Geometry: final body of the model. Coordinates: model frame, mm. A direction names the side the tool comes from. Round coordinates to 2 decimals unless told otherwise and drop trailing zeros. Write each loop counter-clockwise with the first axis right and the second up, starting at its lowest first coordinate (ties: lowest second). Pieces come first, ordered by that corner, then holes.
from build123d import *

# Parameters (mm, degrees)
F4_D            = 6.096
F4_CBORE_D      = 12.192
F4_CBORE_DEPTH  = 6.096
F4_COPIES_COUNT = 6
F5_R            = 7.3585229381
F6_R            = 8.8302275257
F7_SIZE         = 1.27


# Not quite as in the source:
# - a pattern or mirror of a feature is missing from the dataset's text; its kind, count and spacing are read off the source's solid


with BuildPart() as f2:
    # F1 (on Top) → F2 (revolve)
    with BuildSketch(Plane.XY):
        Polygon((0, 23.1950208545), (0, 0), (19.8225509375, 0), (19.8225509375, 20.0292905793), (51.67459324, 20.0292905793), (51.67459324, 28.776070103), (10.3429872543, 28.776070103), (10.3429872543, 23.1950208545), align=None)
    revolve(axis=Axis((0, 11.5975104272, 0), (0, -1, 0)))

    # F4 (through all)
    with Locations(Plane(origin=(0, 28.776070103, 0), x_dir=(-1, 0, 0), z_dir=(0, 1, 0))):
        with Locations((0, -38.1)):
            f4 = CounterBoreHole(F4_D / 2, F4_CBORE_D / 2, F4_CBORE_DEPTH)

    # F4_copies: F4 ×6 about axis
    f4_copies_axis = Axis((0, 0, 0), (0, 1, 0))
    for i in range(1, F4_COPIES_COUNT):
        add(f4.rotate(f4_copies_axis, i * 360 / F4_COPIES_COUNT), mode=Mode.SUBTRACT)

    # F5
    f5_edges = [f2.edges().sort_by_distance(p)[0] for p in [
        (-19.822551, 20.029291, 0),
    ]]
    fillet(f5_edges, radius=F5_R)

    # F6
    f6_edges = [f2.edges().sort_by_distance(p)[0] for p in [
        (-19.822551, 0, 0),
    ]]
    fillet(f6_edges, radius=F6_R)

    # F7
    f7_edges = [f2.edges().sort_by_distance(p)[0] for p in [
        (-51.674593, 20.029291, 0),
        (-51.674593, 28.77607, 0),
    ]]
    chamfer(f7_edges, length=F7_SIZE)


solid = f2.part
1) Section B-B on y = 26.25. Output: boundary loops of the cut face in (x, z), plus the area to 3 significant figures.
2) Section C-C on x = 0. State how many separate pieces and enclosed holes the cut face has, plus the area to 3 significant figures.
3) Line query: probe 1 along Z at (x, y) = (0, 21.8); probe 2 along Z at (x, y) = (0, 26.5); probe 3 along Z at (x, y) = (30, 25.5). Output: solid intervals per line, ascending.
4) Draft query along Z for faces 1 (the cylindrical face through (49.29, 24.45, 15.52)), 2 (the flat face through (-22, 20.029, -22)), 3 (the cylindrical face through (-38.81, 25.77, 20.88)). Return one class per face: pulls with the +Z half, pulls with the -Z half, needs draft (parallel to the pull), parting line crosses it, or undercut.
5) First-contact query: P1, Ø10, axis at x = -25, z = 25.5, coming from the -Y side; P2, Ø12, axis at y = 21.5, z = -28.5, coming from the +X side; P3, Ø6, axis at x = 30.5, z = -20.5, coming from the +Y side. Flat tips, straight axial feed; report the tip coordinate or a pass-through.
6) Reachability of faces 4 (the cylindrical face through (10.66, 10.78, 16.71)), 5 (the flat face through (0, 0, 0)), 6 (the flat face through (30, 22.68, 21)) from +Z, -Z, +X, -X, +Y, -Y: full face, straight path, thin tool, end or side. Return the list, or none.
7) Section A-A on z = 0. Output: boundary loops of the cut face in (x, y).
Filled in:
1. outline: circle Ø103.35 at (0, 0); hole circle Ø12.19 at (-33, -19.05); hole circle Ø12.19 at (-33, 19.05); hole circle Ø20.69 at (0, 0); hole circle Ø12.19 at (0, -38.1); hole circle Ø12.19 at (0, 38.1); hole circle Ø12.19 at (33, -19.05); hole circle Ø12.19 at (33, 19.05)
1. area: 7,350 mm2
2. separate pieces: 3
2. enclosed holes: 0
2. area: 1,390 mm2
3. probe 1: z = -51.67 to -41.15, -35.05 to 35.05, 41.15 to 51.67
3. probe 2: z = -51.67 to -44.2, -32 to -10.34, 10.34 to 32, 44.2 to 51.67
3. probe 3: z = -42.07 to -24.36, -13.74 to 13.74, 24.36 to 42.07
4. face 1: parting line crosses it
4. face 2: needs draft
4. face 3: undercut
5. P1: stops at y = 20.03
5. P2: stops at x = 46.52
5. P3: stops at y = 22.68
6. face 4: -Y
6. face 5: +Z, -Z, +X, -X, -Y
6. face 6: +Y
7. outline: (-51.67, 21.3) - (-50.4, 20.03) - (-27.18, 20.03) arc R7.36 cw to (-19.82, 12.67) - (-19.82, 8.83) arc R8.83 ccw to (-10.99, 0) - (10.99, 0) arc R8.83 ccw to (19.82, 8.83) - (19.82, 12.67) arc R7.36 cw to (27.18, 20.03) - (50.4, 20.03) - (51.67, 21.3) - (51.67, 27.51) - (50.4, 28.78) - (10.34, 28.78) - (10.34, 23.2) - (-10.34, 23.2) - (-10.34, 28.78) - (-50.4, 28.78) - (-51.67, 27.51) - close
